```python
from build123d import *

# Parameters (mm, degrees)
RESSALTO_EXTRUS_O1_DEPTH = 32
FILETE1_R                = 0.2
ESBO_O2_R                = 1.0922
RESSALTO_EXTRUS_O2_DEPTH = 4.76
ESBO_O3_R                = 1.0922
CORTE_EXTRUS_O1_DEPTH    = 4.76


with BuildPart() as part:
    # Esboço1 → Ressalto-extrusão1 (new body)
    with BuildSketch(Plane(origin=(0, 0, 0), x_dir=(1, 0, 0), z_dir=(0, 1, 0))):
        Polygon((2.748187281, 0), (1.374093641, 2.38), (-1.374093641, 2.38), (-2.748187281, 0), (-1.374093641, -2.38), (1.374093641, -2.38), align=None)
    extrude(amount=RESSALTO_EXTRUS_O1_DEPTH)

    # Filete1
    filete1_edges = [part.edges().sort_by_distance(p)[0] for p in [
        (0, 32, -2.38),
        (-2.061140461, 32, -1.19),
        (-2.061140461, 32, 1.19),
        (0, 32, 2.38),
        (2.061140461, 32, 1.19),
        (0, 0, 2.38),
        (-2.061140461, 0, 1.19),
        (-2.061140461, 0, -1.19),
        (2.061140461, 32, -1.19),
        (0, 0, -2.38),
        (2.061140461, 0, -1.19),
        (2.061140461, 0, 1.19),
    ]]
    fillet(filete1_edges, radius=FILETE1_R)

    # Esboço2 → Ressalto-extrusão2 (add)
    with BuildSketch(Plane.XZ):
        Circle(ESBO_O2_R)
    extrude(amount=RESSALTO_EXTRUS_O2_DEPTH)

    # Esboço3 → Corte-extrusão1 (cut)
    with BuildSketch(Plane(origin=(0, 32, 0), x_dir=(1, 0, 0), z_dir=(0, 1, 0))):
        Circle(ESBO_O3_R)
    extrude(amount=-CORTE_EXTRUS_O1_DEPTH, mode=Mode.SUBTRACT)


solid = part.part
```
CAD build for the part. Positions are in the model's coordinates, mm. A direction names the side the tool comes from. Give positions to 0.01 mm unless a question says otherwise; leave off trailing zeros. Write each loop counter-clockwise with the first axis right and the second up, starting at its lowest first coordinate (ties: lowest second). Pieces come first, ordered by that corner, then holes. Notation, with made-up numbers: M 23.25,27.5 L 58.25,27.5 A19 cw 58.25,36.5 Z; hole C 62,50 d3. An arc over 180 degrees is marked long. Return JSON: item names as keys, results as strings. Group by question number.
(1) Band-saw the part on B-B (y = 10). Give the cut face in (x, z), and give its area (3 significant figures).
(2) Mould opens along X. For faces 4 (the face through (1.04, 29.65, -0.33)), 5 (the face through (2.021, 0.06, 1.145)), 6 (the face through (0, 16, -2.38)) say: pulls with the +X half, pulls with the -X half, needs draft (parallel to the pull), parting line crosses it, or undercut.
(3) Drill centre lines: L1, parallel to Z at x = 0, y = 29.55; L2, parallel to Y at x = 1.3, z = 0.55; L3, parallel to Z at x = 1.8, y = 2.5. Where is each one in solid material? Low to high. Write a range as [from, to].
(4) 3-axis set-ups, long thin cutter, end or side, ignore diameter. For faces 1 (the face through (0, 27.24, 0)), 2 (the face through (0, -4.76, 0)), 3 (the face through (1, 0, -1)): which of +Z, -Z, +X, -X, +Y, -Y reach the whole face in a straight line?
(5) Flat gauge pins, fed straight in: pin 1 Ø1 at (x, z) = (1.5, -1.5) entering from -Y; pin 2 Ø2 at (x, z) = (0, 0) entering from +Y. Where does each tip first touch, or does it go through?
(6) Band-saw the part on A-A (x = 0). Give the cut face in (y, z).
Entries:
{
 "1": {"outline": "M -2.75,0 L -1.37,-2.38 L 1.37,-2.38 L 2.75,0 L 1.37,2.38 L -1.37,2.38 Z", "area": "19.6 mm^2"},
 "2": {"face 4": "undercut", "face 5": "pulls with the +X half", "face 6": "needs draft"},
 "3": {"L1": "z = [-2.38, -1.09], [1.09, 2.38]", "L2": "y = [0, 32]", "L3": "z = [-1.64, 1.64]"},
 "4": {"face 1": "+Y", "face 2": "+Z, -Z, +X, -X, -Y", "face 3": "-Y"},
 "5": {"pin 1": "stops at y = 0", "pin 2": "stops at y = 27.24"},
 "6": {"outline": "M -4.76,-1.09 L 0,-1.09 L 0,-2.18 A0.2 ccw 0.2,-2.38 L 31.8,-2.38 A0.2 ccw 32,-2.18 L 32,-1.09 L 27.24,-1.09 L 27.24,1.09 L 32,1.09 L 32,2.18 A0.2 ccw 31.8,2.38 L 0.2,2.38 A0.2 ccw 0,2.18 L 0,1.09 L -4.76,1.09 Z"}
}
